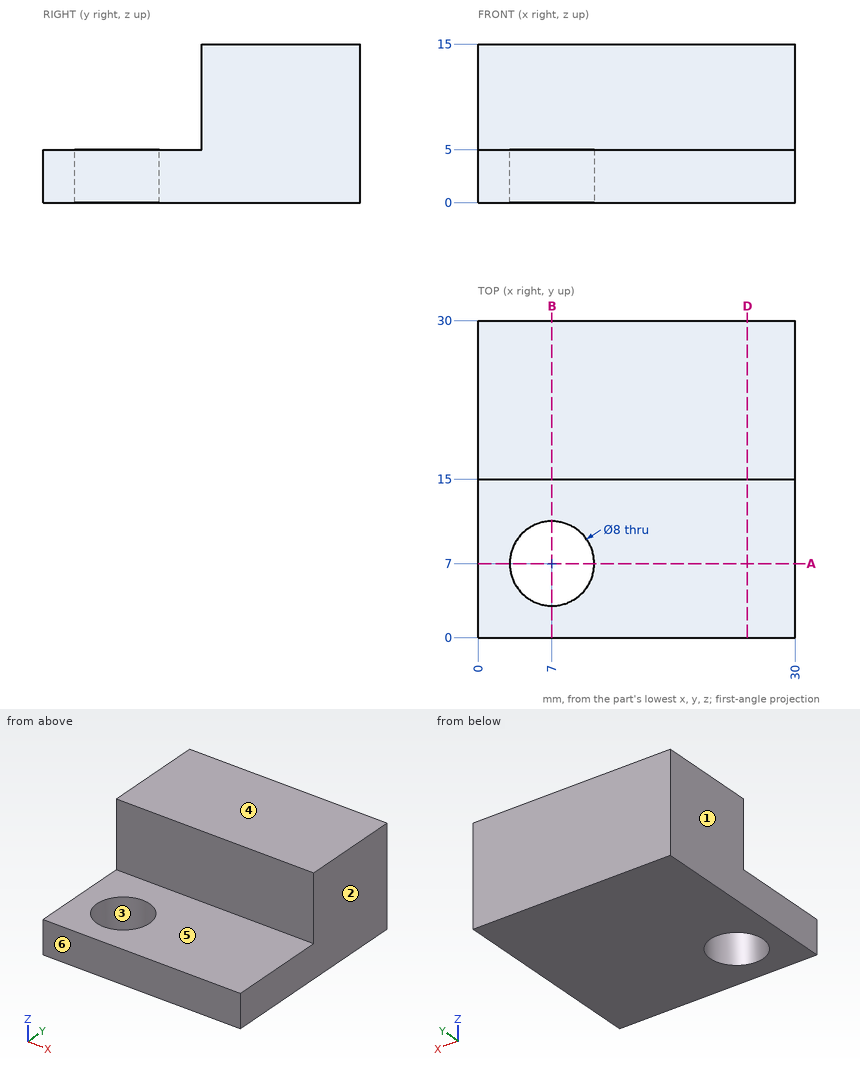
Drawing for the job (mm, zero at the part's lowest x, y, z). A direction names the side the tool comes from. Coordinates: 2 decimals unless noted, no trailing zeros. Loops run counter-clockwise (first coordinate to the right, second up) from the corner with the lowest first, then second, coordinate; pieces in that order, holes last. Notation, with made-up numbers: (-2, 6.5) - (47, 6.5) arc R16 cw to (47, 12.5) - close; hole circle Ø3 at (45.25, 12). An arc over 180 degrees is marked (long way). Return JSON: item names as keys, results as strings.
1. Band-saw the part on A-A (y = 7). Give the cut face in (x, z), and give its area (3 significant figures).
Result:
{"outline": "(0, 0) - (3, 0) - (3, 5) - (0, 5) - close; (11, 0) - (30, 0) - (30, 5) - (11, 5) - close", "area": "110 mm2"}
2. Band-saw the part on D-D (x = 25.5). Give the cut face in (y, z), and give its area (3 significant figures).
Result:
{"outline": "(0, 0) - (30, 0) - (30, 15) - (15, 15) - (15, 5) - (0, 5) - close", "area": "300 mm2"}
3. Probe L1, parallel to Y at x = 7, z = 3.1; L2, parallel to Z at x = 6.25, y = 2.5; L3, parallel to X at y = 5.25, z = 1.25. List the from-to ranges inside material, lowest first. Write a range as from..to.
Result:
{"L1": "y = 0..3, 11..30", "L2": "z = 0..5", "L3": "x = 0..3.4, 10.6..30"}
4. Band-saw the part on B-B (x = 7). Give the cut face in (y, z), and give its area (3 significant figures).
Result:
{"outline": "(0, 0) - (3, 0) - (3, 5) - (0, 5) - close; (11, 0) - (30, 0) - (30, 15) - (15, 15) - (15, 5) - (11, 5) - close", "area": "260 mm2"}
5. 3-axis set-ups, long thin cutter, end or side, ignore diameter. For the marked faces 5 and 6: which of +Z, -Z, +X, -X, +Y, -Y reach the whole face in a straight line?
Result:
{"face 5": "+Z, +X, -X, -Y", "face 6": "+Z, -Z, +X, -X, -Y"}
6. Drop flat-ended pins along their axis: pin 1 (2 mm diameter, centred on x = 21, z = 11.5, fed in from -Y); pin 2 (12 mm diameter, centred on x = 12, y = 7, fed in from +Z). Give the stop position or say it passes through.
Result:
{"pin 1": "stops at y = 15", "pin 2": "stops at z = 5"}
7. Mould opens along X. For the marked faces 1, 2, 3 and 4 say: released by +X, released by -X, zero draft, split by the parting line, or undercut.
Result:
{"face 1": "released by -X", "face 2": "released by +X", "face 3": "undercut", "face 4": "zero draft"}
